```python
from build123d import *

# Parameters (mm, degrees)
F0_R     = 50.8
F1_DEPTH = 6.35


with BuildPart() as f1:
    # F0 (on Front) → F1 (new body, symmetric)
    with BuildSketch(Plane.XZ):
        with BuildLine():
            ThreePointArc((-58.42, 0), (0, -58.42), (58.42, 0))
            ThreePointArc((58.42, 0), (41.309178, 41.309178), (0, 58.42))
            ThreePointArc((0, 58.42), (-41.309178, 41.309178), (-58.42, 0))
        make_face()
        Circle(F0_R, mode=Mode.SUBTRACT)
        with BuildLine():
            ThreePointArc((-58.42, 0), (-41.309178, 41.309178), (0, 58.42))
            ThreePointArc((0, 58.42), (-6.348121, 60.647349), (-9.91288, 66.352804))
            ThreePointArc((-9.91288, 66.352804), (-45.000104, 41.096336), (-58.42, 0))
        make_face()
    extrude(amount=F1_DEPTH, both=True)

    # F2 (on Right) → F3 (revolve)
    with BuildSketch(Plane.YZ):
        with BuildLine():
            Line((6.35, 50.8), (-6.35, 50.8))
            ThreePointArc((-6.35, 50.8), (0, 49.53), (6.35, 50.8))
        make_face()
    revolve(axis=Axis((0, 1.744404, 0), (0, 1, 0)))


solid = f1.part
```
Read the model definition and answer for the solid it produces. Units are mm, in the model's axes. Give positions to 0.01 mm unless a question says otherwise; leave off trailing zeros. Order: outer loops, then holes, each group sorted by start corner. A loop starts at its lowest first (then second) coordinate and runs counter-clockwise, first axis right, second up. Notation, with made-up numbers: (-1.5, -25.75) -> (26.5, -25.75) arc R38 ccw to (26.5, 12.25) -> close; hole circle Ø11 at (31.25, -33.75). An arc over 180 degrees is marked (long way). Write item = value, one per line.
1. A cutting plane is placed at A-A, the plane y = 4. Write down the section's boundary in (x, z), and give its area (3 significant figures).
Numbers:
outline = (-58.42, 0) arc R58.42 ccw (long way) to (0, 58.42) arc R10.16 cw to (-9.91, 66.35) arc R69.64 ccw to start; hole circle Ø100.04 at (0, 0)
area = 3,140 mm²
2. Straight lines are drawn through the part: line 1 along Z through (x, y) = (-40.5, -4.25); line 2 along X through (y, z) = (-3, 9.5); line 3 along X through (y, z) = (4.5, 39). For each, find the intervals that lie inside material, in ascending order.
Numbers:
line_1 = -42.1 to -29.47, 29.47 to 46.63
line_2 = -57.77 to -48.89, 48.89 to 57.64
line_3 = -46.47 to -31.54, 31.54 to 43.5
3. Given pin 1 (4 mm diameter, centred on y = -2.5, z = 12, fed in from -X); pin 2 (4 mm diameter, centred on x = 32.5, y = 2, fed in from +Z); pin 3 (4 mm diameter, centred on x = -10, y = 2, fed in from -Z), each flat-ended and moving along its own axis, determine where each tip first touches the part or whether it passes through.
Numbers:
pin_1 = -57.7
pin_2 = 49.83
pin_3 = -57.87
